```python
from build123d import *


with BuildPart() as f3:
    # F3: sweep along a path in F0
    with BuildLine(Plane.XY) as f3_path:
        Line((0, -67), (0, -5))
        ThreePointArc((0, -5), (1.464466, -1.464466), (5, 0))
        Line((5, 0), (25, 0))
    # F2 (on face) → F3 (sweep)
    with BuildSketch(Plane(origin=(0, -67, 0), x_dir=(-1, 0, 0), z_dir=(0, 1, 0))):
        Polygon((-1.059994, 2.051766), (-2.306879, 0.107901), (-1.246885, -1.943865), (1.059994, -2.051766), (2.306879, -0.107901), (1.246885, 1.943865), align=None)
    sweep(path=f3_path.line)


solid = f3.part
```
Model file for the job. Use its own axes, mm. A direction names the side the tool comes from. Round coordinates to 2 decimals unless told otherwise and drop trailing zeros. Order: outer loops, then holes, each group sorted by start corner. A loop starts at its lowest first (then second) coordinate and runs counter-clockwise, first axis right, second up. Notation, with made-up numbers: (46, -31.5) -> (51, -31.5) arc R20 ccw to (51, -21.5) -> close; hole circle Ø8 at (11, 24). An arc over 180 degrees is marked (long way). Use one line per item in the form item = value.
Item 1: Tool access for faces 1 (the face through (1.675, -35.566, 1.093)), 2 (the face through (15.14, -0.11, -1.997)), 3 (the face through (-1.675, -35.566, -1.093)): list every direction of +Z, -Z, +X, -X, +Y, -Y with a clear straight run to the whole face (end or side of a thin tool).
Returned:
face_1 = +Z, +X, -Y
face_2 = -Z, +X, -Y
face_3 = -Z, -X, +Y, -Y
Item 2: Flat gauge pin, fed straight in: pin 1 Ø10 at (x, y) = (2, -23.5) entering from +Z. Where does the tip first touch, or does it go through?
Returned:
pin_1 = 2.05
Item 3: Cut at A-A, the plane y = -52. Write the cut outline in (x, z).
Returned:
outline = (-2.31, -0.11) -> (-1.06, -2.05) -> (1.25, -1.94) -> (2.31, 0.11) -> (1.06, 2.05) -> (-1.25, 1.94) -> close
Item 4: Cut at B-B, the plane z = -0.75. Write the cut outline in (x, y) (3 decimals).
Returned:
outline = (-1.895, -67) -> (1.864, -67) -> (1.864, -5) arc R3.136 cw to (5, -1.864) -> (25, -1.864) -> (25, 1.895) -> (5, 1.895) arc R6.895 ccw to (-1.895, -5) -> close
Item 5: Drill centre lines: line 1 (X direction, y = -6, z = -0.05); line 2 (Z direction, x = 2.25, y = -6.5); line 3 (Y direction, x = 3.5, z = -1.75). Where is each one in solid material? Low to high.
Returned:
line_1 = -2.28 to 2.23
line_2 = 0 to 0.2
line_3 = -1.67 to 1.07
Item 6: Cut at C-C, the plane x = 22. Write the cut outline in (y, z).
Returned:
outline = (-2.31, 0.11) -> (-1.25, -1.94) -> (1.06, -2.05) -> (2.31, -0.11) -> (1.25, 1.94) -> (-1.06, 2.05) -> close
